For this review, take the finished solid that the model builds, in its own axes (mm). A direction names the side the tool comes from. Round coordinates to 2 decimals unless told otherwise and drop trailing zeros. Write each loop counter-clockwise with the first axis right and the second up, starting at its lowest first coordinate (ties: lowest second). Pieces come first, ordered by that corner, then holes. Notation, with made-up numbers: M 73.5,-27 L 97.5,-27 A6 ccw 97.5,-22 Z; hole C 61.5,67 d4. An arc over 180 degrees is marked long. One line per question, with ' | ' between items.
```python
from build123d import *

# Parameters (mm, degrees)
EXTRUDE_4_DEPTH = 10


with BuildPart() as part:
    # 草圖1 → 填料-伸長4 (new body)
    with BuildSketch(Plane.XY):
        Polygon((49.802669845, 25.924393386), (-10.397330155, 25.924393386), (-29.457330155, -7.088495007), (0.642669845, -59.223224314), (38.762669845, -59.223224314), (68.862669845, -7.088495007), align=None)
        with BuildLine():
            Line((-0.037670798, 33.71862202), (-3.897330155, 33.71862202))
            ThreePointArc((-3.897330155, 33.71862202), (-4.897330155, 31.986571212), (-6.897330155, 31.986571212))
            Line((-6.897330155, 31.986571212), (-10.397330155, 25.924393386))
            Line((-10.397330155, 25.924393386), (49.802669845, 25.924393386))
            Line((49.802669845, 25.924393386), (46.302669845, 31.986571212))
            ThreePointArc((46.302669845, 31.986571212), (44.302669845, 31.986571212), (43.302669845, 33.71862202))
            Line((43.302669845, 33.71862202), (39.302669845, 33.71862202))
            ThreePointArc((39.302669845, 33.71862202), (37.302669845, 31.71862202), (35.302669845, 33.71862202))
            Line((35.302669845, 33.71862202), (31.302669845, 33.71862202))
            ThreePointArc((31.302669845, 33.71862202), (29.302669845, 31.71862202), (27.302669845, 33.71862202))
            Line((27.302669845, 33.71862202), (12.102669845, 33.71862202))
            ThreePointArc((12.102669845, 33.71862202), (10.102669845, 31.71862202), (8.102669845, 33.71862202))
            Line((8.102669845, 33.71862202), (3.962329202, 33.71862202))
            ThreePointArc((3.962329202, 33.71862202), (1.962329202, 31.71862202), (-0.037670798, 33.71862202))
        make_face()
        with BuildLine():
            ThreePointArc((-6.897330155, 31.986571212), (-6.897330155, 35.450672827), (-3.897330155, 33.71862202))
            Line((-3.897330155, 33.71862202), (-0.037670798, 33.71862202))
            ThreePointArc((-0.037670798, 33.71862202), (1.962329202, 35.71862202), (3.962329202, 33.71862202))
            Line((3.962329202, 33.71862202), (8.102669845, 33.71862202))
            ThreePointArc((8.102669845, 33.71862202), (10.102669845, 35.71862202), (12.102669845, 33.71862202))
            Line((12.102669845, 33.71862202), (27.302669845, 33.71862202))
            ThreePointArc((27.302669845, 33.71862202), (29.302669845, 35.71862202), (31.302669845, 33.71862202))
            Line((31.302669845, 33.71862202), (35.302669845, 33.71862202))
            ThreePointArc((35.302669845, 33.71862202), (37.302669845, 35.71862202), (39.302669845, 33.71862202))
            Line((39.302669845, 33.71862202), (43.302669845, 33.71862202))
            ThreePointArc((43.302669845, 33.71862202), (45.302669845, 35.71862202), (47.302669845, 33.71862202))
            ThreePointArc((47.302669845, 33.71862202), (47.034720652, 32.71862202), (46.302669845, 31.986571212))
            Line((46.302669845, 31.986571212), (49.802669845, 25.924393386))
            Line((49.802669845, 25.924393386), (49.802669845, 37.924393386))
            Line((49.802669845, 37.924393386), (-10.397330155, 37.924393386))
            Line((-10.397330155, 37.924393386), (-10.397330155, 25.924393386))
            Line((-10.397330155, 25.924393386), (-6.897330155, 31.986571212))
        make_face()
        with BuildLine():
            Line((-32.957330155, -13.150672833), (-29.457330155, -7.088495007))
            Line((-29.457330155, -7.088495007), (-39.849635001, -13.088495007))
            Line((-39.849635001, -13.088495007), (-9.749635001, -65.223224314))
            Line((-9.749635001, -65.223224314), (0.642669845, -59.223224314))
            Line((0.642669845, -59.223224314), (-6.357330155, -59.223224314))
            ThreePointArc((-6.357330155, -59.223224314), (-9.357330155, -60.955275122), (-9.357330155, -57.491173507))
            Line((-9.357330155, -57.491173507), (-11.357330155, -54.027071892))
            ThreePointArc((-11.357330155, -54.027071892), (-14.089380963, -53.295021084), (-13.357330155, -50.562970277))
            Line((-13.357330155, -50.562970277), (-15.394263476, -47.034898273))
            ThreePointArc((-15.394263476, -47.034898273), (-18.229721605, -46.366817854), (-17.390567155, -43.577198874))
            Line((-17.390567155, -43.577198874), (-24.994263476, -30.40721052))
            ThreePointArc((-24.994263476, -30.40721052), (-27.829721605, -29.739130101), (-26.990567155, -26.949511121))
            Line((-26.990567155, -26.949511121), (-28.994263476, -23.47900729))
            ThreePointArc((-28.994263476, -23.47900729), (-31.829721605, -22.810926871), (-30.990567155, -20.021307891))
            Line((-30.990567155, -20.021307891), (-32.957330155, -16.614774448))
            ThreePointArc((-32.957330155, -16.614774448), (-35.957330155, -14.882723641), (-32.957330155, -13.150672833))
        make_face()
        with BuildLine():
            Line((0.642669845, -59.223224314), (-29.457330155, -7.088495007))
            Line((-29.457330155, -7.088495007), (-32.957330155, -13.150672833))
            ThreePointArc((-32.957330155, -13.150672833), (-32.225279348, -13.882723641), (-31.957330155, -14.882723641))
            ThreePointArc((-31.957330155, -14.882723641), (-32.225279348, -15.882723641), (-32.957330155, -16.614774448))
            Line((-32.957330155, -16.614774448), (-30.990567155, -20.021307891))
            ThreePointArc((-30.990567155, -20.021307891), (-29.045480871, -20.110075214), (-28.097670798, -21.810926871))
            ThreePointArc((-28.097670798, -21.810926871), (-28.336021763, -22.75781265), (-28.994263476, -23.47900729))
            Line((-28.994263476, -23.47900729), (-26.990567155, -26.949511121))
            ThreePointArc((-26.990567155, -26.949511121), (-25.045480871, -27.038278445), (-24.097670798, -28.739130101))
            ThreePointArc((-24.097670798, -28.739130101), (-24.336021763, -29.68601588), (-24.994263476, -30.40721052))
            Line((-24.994263476, -30.40721052), (-17.390567155, -43.577198874))
            ThreePointArc((-17.390567155, -43.577198874), (-15.445480871, -43.665966197), (-14.497670798, -45.366817854))
            ThreePointArc((-14.497670798, -45.366817854), (-14.736021763, -46.313703633), (-15.394263476, -47.034898273))
            Line((-15.394263476, -47.034898273), (-13.357330155, -50.562970277))
            ThreePointArc((-13.357330155, -50.562970277), (-11.357330155, -50.562970277), (-10.357330155, -52.295021084))
            ThreePointArc((-10.357330155, -52.295021084), (-10.625279348, -53.295021084), (-11.357330155, -54.027071892))
            Line((-11.357330155, -54.027071892), (-9.357330155, -57.491173507))
            ThreePointArc((-9.357330155, -57.491173507), (-7.357330155, -57.491173507), (-6.357330155, -59.223224314))
            Line((-6.357330155, -59.223224314), (0.642669845, -59.223224314))
        make_face()
        with BuildLine():
            Line((79.25497469, -13.088495007), (68.862669845, -7.088495007))
            Line((68.862669845, -7.088495007), (72.362669845, -13.150672833))
            ThreePointArc((72.362669845, -13.150672833), (74.362669845, -13.150672833), (75.362669845, -14.882723641))
            ThreePointArc((75.362669845, -14.882723641), (74.362669845, -16.614774448), (72.362669845, -16.614774448))
            Line((72.362669845, -16.614774448), (70.362669845, -20.078876063))
            ThreePointArc((70.362669845, -20.078876063), (71.094720652, -20.810926871), (71.362669845, -21.810926871))
            ThreePointArc((71.362669845, -21.810926871), (70.362669845, -23.542977679), (68.362669845, -23.542977679))
            Line((68.362669845, -23.542977679), (66.362669845, -27.007079294))
            ThreePointArc((66.362669845, -27.007079294), (67.094720652, -27.739130101), (67.362669845, -28.739130101))
            ThreePointArc((67.362669845, -28.739130101), (66.362669845, -30.471180909), (64.362669845, -30.471180909))
            Line((64.362669845, -30.471180909), (56.762669845, -43.634767046))
            ThreePointArc((56.762669845, -43.634767046), (57.494720652, -44.366817854), (57.762669845, -45.366817854))
            ThreePointArc((57.762669845, -45.366817854), (56.762669845, -47.098868661), (54.762669845, -47.098868661))
            Line((54.762669845, -47.098868661), (52.762669845, -50.562970277))
            ThreePointArc((52.762669845, -50.562970277), (53.494720652, -51.295021084), (53.762669845, -52.295021084))
            ThreePointArc((53.762669845, -52.295021084), (52.762669845, -54.027071892), (50.762669845, -54.027071892))
            Line((50.762669845, -54.027071892), (48.762669845, -57.491173507))
            ThreePointArc((48.762669845, -57.491173507), (49.494720652, -58.223224314), (49.762669845, -59.223224314))
            ThreePointArc((49.762669845, -59.223224314), (47.762669845, -61.223224314), (45.762669845, -59.223224314))
            Line((45.762669845, -59.223224314), (38.762669845, -59.223224314))
            Line((38.762669845, -59.223224314), (49.15497469, -65.223224314))
            Line((49.15497469, -65.223224314), (79.25497469, -13.088495007))
        make_face()
        with BuildLine():
            Line((72.362669845, -13.150672833), (68.862669845, -7.088495007))
            Line((68.862669845, -7.088495007), (38.762669845, -59.223224314))
            Line((38.762669845, -59.223224314), (45.762669845, -59.223224314))
            ThreePointArc((45.762669845, -59.223224314), (46.762669845, -57.491173507), (48.762669845, -57.491173507))
            Line((48.762669845, -57.491173507), (50.762669845, -54.027071892))
            ThreePointArc((50.762669845, -54.027071892), (50.030619037, -51.295021084), (52.762669845, -50.562970277))
            Line((52.762669845, -50.562970277), (54.762669845, -47.098868661))
            ThreePointArc((54.762669845, -47.098868661), (54.030619037, -44.366817854), (56.762669845, -43.634767046))
            Line((56.762669845, -43.634767046), (64.362669845, -30.471180909))
            ThreePointArc((64.362669845, -30.471180909), (63.630619037, -27.739130101), (66.362669845, -27.007079294))
            Line((66.362669845, -27.007079294), (68.362669845, -23.542977679))
            ThreePointArc((68.362669845, -23.542977679), (67.630619037, -20.810926871), (70.362669845, -20.078876063))
            Line((70.362669845, -20.078876063), (72.362669845, -16.614774448))
            ThreePointArc((72.362669845, -16.614774448), (71.362669845, -14.882723641), (72.362669845, -13.150672833))
        make_face()
    extrude(amount=EXTRUDE_4_DEPTH)


solid = part.part
```
Item 1: Take a section at C-C (y = -1). Write out the cut boundary in (x, z).
Results:
outline: M -25.94,0 L 65.35,0 L 65.35,10 L -25.94,10 Z
Item 2: Take a section at A-A (z = 8). State how many separate pieces and enclosed holes the cut face has, then the cut area to 3 significant figures.
Results:
separate pieces: 1 | enclosed holes: 18 | area: 8,110 mm2
Item 3: To check wall thickness, follow line 1 along X through (y, z) = (-23, 3); line 2 along X through (y, z) = (-30, 6.5); line 3 along Y through (x, z) = (45, 4.25). State the ranges of each line that lie inside material, in increasing order. Write a range as from..to.
Results:
line 1: -34.13..-31.71, -28.49..67.75, 70.97..73.53 | line 2: -30.09..-27.65, -24.55..63.81, 66.92..69.49 | line 3: -62.82..31.74, 35.7..37.92
Item 4: Take a section at B-B (x = 23.5). Write out the cut boundary in (y, z).
Results:
outline: M -59.22,0 L 37.92,0 L 37.92,10 L -59.22,10 Z
Item 5: Mouldability with a two-part tool opening along X and no side actions: class faces 6 (the face through (-25.01, -38.79, 4.93)), 7 (the face through (8.255, 32.953, 4.93)), 8 (the face through (74.13, -10.13, 4.93)) as +X half, -X half, draft (parallel to the pull), parting line (faces both ways), or undercut.
Results:
face 6: -X half | face 7: undercut | face 8: +X half
Item 6: Insertion check: pin 1 Ø2 at (y, z) = (-38.5, 5.5) entering from +X; pin 2 Ø5 at (x, z) = (23.5, 6) entering from -Y; pin 3 Ø5 at (x, y) = (-9.5, -41.5) entering from -Z; pin 4 Ø2.5 at (x, y) = (37.3, 33.72) entering from +Z. Each pin has a flat end and moves straight along its axis. Give the tip position at first contact, or say it passes through.
Results:
pin 1: x = 65.16 | pin 2: y = -59.22 | pin 3: z = 0 | pin 4: through
Item 7: Machinability: for faces 1 (the face through (43.886, -62.181, 4.93)), 2 (the face through (49.803, 32, 5)), 3 (the face through (-10.397, 32, 5)), 4 (the face through (19, -13, 10)), 5 (the face through (35.455, 32.953, 4.93)), which of the approach directions +Z, -Z, +X, -X, +Y, -Y give a long, thin tool a straight path to every point of the face, cutting with its end or side? Answer none if there is none.
Results:
face 1: +Z, -Z, -Y | face 2: +Z, -Z, +X, +Y | face 3: +Z, -Z, -X, +Y | face 4: +Z, +X, -X, +Y, -Y | face 5: +Z, -Z
